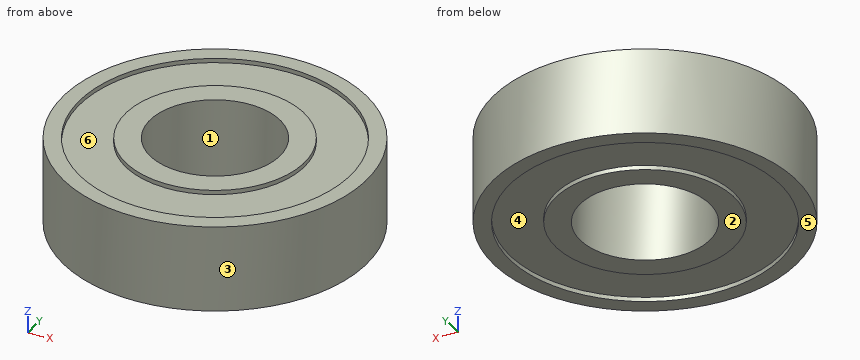
```python
from build123d import *

# Parameters (mm, degrees)
SKETCH1_R          = 14
SKETCH1_R_2        = 6
EXTRUDE1_DEPTH     = 4
SKETCH2_R          = 12.5
SKETCH2_R_2        = 8.25
CUT_EXTRUDE1_DEPTH = 0.4


with BuildPart() as part:
    # Sketch1 → Extrude1 (new, symmetric)
    with BuildSketch(Plane.XY):
        Circle(SKETCH1_R)
        Circle(SKETCH1_R_2, mode=Mode.SUBTRACT)
    extrude(amount=EXTRUDE1_DEPTH, both=True)

    # Sketch2 → Cut-Extrude1 (cut)
    with BuildSketch(Plane.XY.offset(4)):
        Circle(SKETCH2_R)
        Circle(SKETCH2_R_2, mode=Mode.SUBTRACT)
    cut_extrude1 = extrude(amount=-CUT_EXTRUDE1_DEPTH, mode=Mode.SUBTRACT)

    # Mirror1: Cut-Extrude1 across plane
    add(cut_extrude1.mirror(Plane.XY), mode=Mode.SUBTRACT)


solid = part.part
```
The listing builds one solid part. Answer for the finished solid, in the listing's coordinates (mm). Face numbers are marked on the shaded views. A direction names the side the tool comes from. Coordinates: 2 decimals unless noted, no trailing zeros. Order: outer loops, then holes, each group sorted by start corner. A loop starts at its lowest first (then second) coordinate and runs counter-clockwise, first axis right, second up. Notation, with made-up numbers: M -18.75,-4 L -2.75,-4 A13 ccw -2.75,7 Z; hole C 67.25,76 d9. An arc over 180 degrees is marked long. Answer as a JSON object with one key per item and string values. Group by question number.
1. Section D-D on z = 1.5 is taken. Write down the section's boundary in (x, y), then the cut area to 3 significant figures.
2. A tool of negligible diameter and unlimited length cuts with its end or side. For the marked faces 4, 5 and 6, from which of +Z, -Z, +X, -X, +Y, -Y can it reach the whole face along a straight path? Write none if from no direction.
3. Section A-A on y = 0 is taken. Write down the section's boundary in (x, z).
4. Straight lines are drawn through the part: line 1 (Y direction, x = 0, z = -3.9); line 2 (Y direction, x = 0.25, z = 0.75). For each, find the intervals that lie inside material, in ascending order.
5. Section C-C on x = 7.5 is taken. Write down the section's boundary in (y, z), then the cut area to 3 significant figures.
6. Flat-ended cylindrical pins translate along their axes: P1, Ø1.5, axis at x = 7, z = 2, coming from the +Y side; P2, Ø3, axis at y = 2.5, z = -3, coming from the +X side; P3, Ø9.5, axis at x = 0, y = 0, coming from the +Z side; P4, Ø2, axis at x = 5, z = 1, coming from the +Y side. Find the tip coordinate at first contact, or state that the pin passes through.
7. Determine the mould class of the marked faces 1, 2 and 3 for opening direction X: released by +X, released by -X, zero draft, split by the parting line, or undercut.
Values follow:
{
 "1": {"outline": "C 0,0 d28; hole C 0,0 d12", "area": "503 mm2"},
 "2": {"face 4": "-Z", "face 5": "-Z, +X, -X, +Y, -Y", "face 6": "+Z"},
 "3": {"outline": "M -14,-4 L -12.5,-4 L -12.5,-3.6 L -8.25,-3.6 L -8.25,-4 L -6,-4 L -6,4 L -8.25,4 L -8.25,3.6 L -12.5,3.6 L -12.5,4 L -14,4 Z; M 6,-4 L 8.25,-4 L 8.25,-3.6 L 12.5,-3.6 L 12.5,-4 L 14,-4 L 14,4 L 12.5,4 L 12.5,3.6 L 8.25,3.6 L 8.25,4 L 6,4 Z"},
 "4": {"line 1": "-14 to -12.5, -8.25 to -6, 6 to 8.25, 12.5 to 14", "line 2": "-14 to -5.99, 5.99 to 14"},
 "5": {"outline": "M -11.82,-4 L -10,-4 L -10,-3.6 L -3.44,-3.6 L -3.44,-4 L 3.44,-4 L 3.44,-3.6 L 10,-3.6 L 10,-4 L 11.82,-4 L 11.82,4 L 10,4 L 10,3.6 L 3.44,3.6 L 3.44,4 L -3.44,4 L -3.44,3.6 L -10,3.6 L -10,4 L -11.82,4 Z", "area": "179 mm2"},
 "6": {"P1": "y = 12.53", "P2": "x = 13.96", "P3": "through", "P4": "y = 13.42"},
 "7": {"face 1": "undercut", "face 2": "zero draft", "face 3": "split by the parting line"}
}
